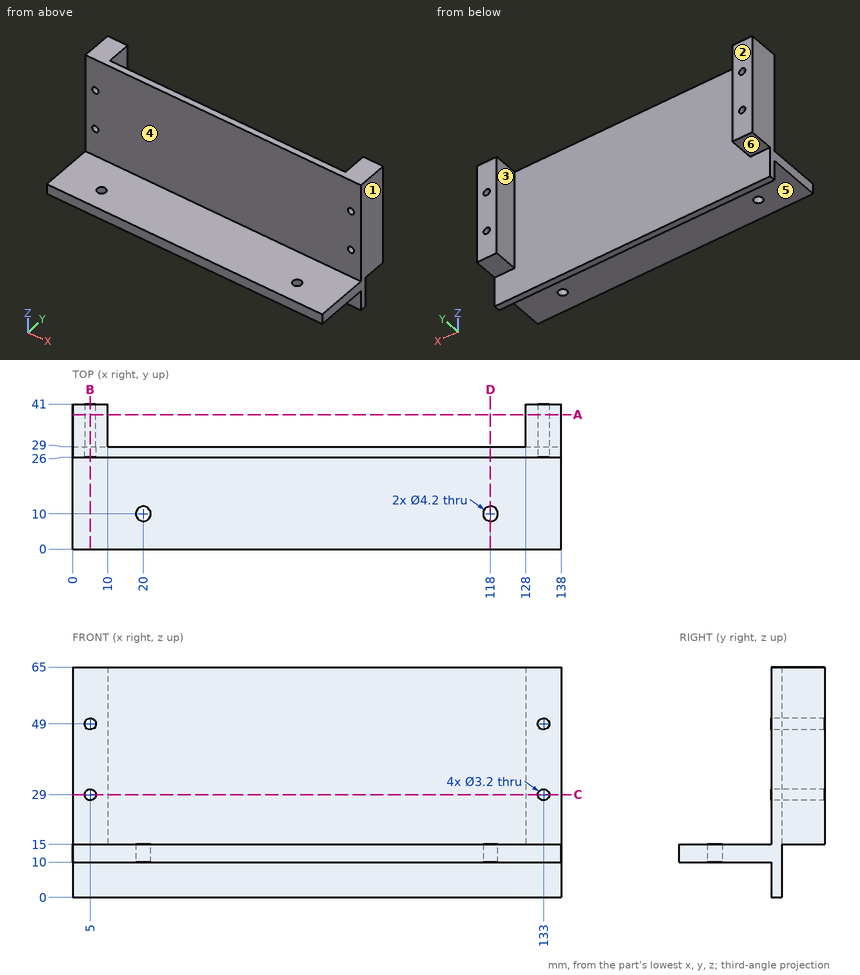
Input: dimensioned drawing with shaded views. Units: mm. Origin: part minimum x, y, z. A direction names the side the tool comes from. Give positions to 0.01 mm unless a question says otherwise; leave off trailing zeros. Loops run counter-clockwise (first coordinate to the right, second up) from the corner with the lowest first, then second, coordinate; pieces in that order, holes last. Notation, with made-up numbers: (20.25, -15) -> (44.25, -15) arc R21 ccw to (44.25, 7) -> close; hole circle Ø2 at (-13.5, 17). An arc over 180 degrees is marked (long way). Use a Markdown table: item, result.
Q1. Section query C-C, the plane z = 29. Return the cut outline in (x, y), plus the area to 3 significant figures.
Entries:
| item | result |
|---|---|
| outline | (0, 26) -> (3.4, 26) -> (3.4, 41) -> (0, 41) -> close; (6.6, 26) -> (131.4, 26) -> (131.4, 41) -> (128, 41) -> (128, 29) -> (10, 29) -> (10, 41) -> (6.6, 41) -> close; (134.6, 26) -> (138, 26) -> (138, 41) -> (134.6, 41) -> close |
| area | 558 mm² |
Q2. First-contact query: P1, Ø5, axis at x = 5, z = 49, coming from the -Y side; P2, Ø12, axis at x = 48.5, y = 11, coming from the +Z side; P3, Ø12, axis at x = 77.5, z = 49, coming from the +Y side; P4, Ø5, axis at x = 5, z = 29, coming from the +Y side. Flat tips, straight axial feed; report the tip coordinate or a pass-through.
Entries:
| item | result |
|---|---|
| P1 | stops at y = 26 |
| P2 | stops at z = 15 |
| P3 | stops at y = 29 |
| P4 | stops at y = 41 |
Q3. Access query for the marked faces 4, 5 and 6. Directions: +Z, -Z, +X, -X, +Y, -Y. A direction counts if a zero-diameter tool reaches every point of the face in a straight line with its end or side. Return the directions, or none.
Entries:
| item | result |
|---|---|
| face 4 | +Z, +X, -X, -Y |
| face 5 | -Z, +X, -X, -Y |
| face 6 | -Z, +X, -X, +Y |
Q4. Ray query, probe 1 along Z at (x, y) = (133, 29.5); probe 2 along X at (y, z) = (34.25, 49); probe 3 along X at (y, z) = (30, 31.5). Return the intervals inside material, ascending. Write a range as from..to.
Entries:
| item | result |
|---|---|
| probe 1 | z = 15..27.4, 30.6..47.4, 50.6..65 |
| probe 2 | x = 0..3.4, 6.6..10, 128..131.4, 134.6..138 |
| probe 3 | x = 0..10, 128..138 |
Q5. Section query B-B, the plane x = 5. Return the cut outline in (y, z), plus the area to 3 significant figures.
Entries:
| item | result |
|---|---|
| outline | (0, 10) -> (26, 10) -> (26, 0) -> (29, 0) -> (29, 15) -> (41, 15) -> (41, 27.4) -> (26, 27.4) -> (26, 15) -> (0, 15) -> close; (26, 30.6) -> (41, 30.6) -> (41, 47.4) -> (26, 47.4) -> close; (26, 50.6) -> (41, 50.6) -> (41, 65) -> (26, 65) -> close |
| area | 829 mm² |
Q6. Pull-direction query (X, two-part tool) for the marked faces 1, 2 and 3; classes: pulls with the +X half, pulls with the -X half, needs draft (parallel to the pull), parting line crosses it, or undercut.
Entries:
| item | result |
|---|---|
| face 1 | pulls with the +X half |
| face 2 | needs draft |
| face 3 | undercut |
Q7. Section query A-A, the plane y = 38. Return the cut outline in (x, z).
Entries:
| item | result |
|---|---|
| outline | (0, 15) -> (10, 15) -> (10, 65) -> (0, 65) -> close; (128, 15) -> (138, 15) -> (138, 65) -> (128, 65) -> close; hole circle Ø3.2 at (5, 29); hole circle Ø3.2 at (5, 49); hole circle Ø3.2 at (133, 29); hole circle Ø3.2 at (133, 49) |
Q8. Section query D-D, the plane x = 118. Return the cut outline in (y, z).
Entries:
| item | result |
|---|---|
| outline | (0, 10) -> (7.9, 10) -> (7.9, 15) -> (0, 15) -> close; (12.1, 10) -> (26, 10) -> (26, 0) -> (29, 0) -> (29, 65) -> (26, 65) -> (26, 15) -> (12.1, 15) -> close |
